Could you check a few things on this model? Use its own coordinates, in mm. Face numbers are marked on the shaded views. A direction names the side the tool comes from. Round coordinates to 2 decimals unless told otherwise and drop trailing zeros. Loops run counter-clockwise (first coordinate to the right, second up) from the corner with the lowest first, then second, coordinate; pieces in that order, holes last. Notation, with made-up numbers: (26, 2) -> (43, 2) arc R15 cw to (43, 27) -> close; hole circle Ø7 at (51, 10). An arc over 180 degrees is marked (long way). One line per item, written item: value.
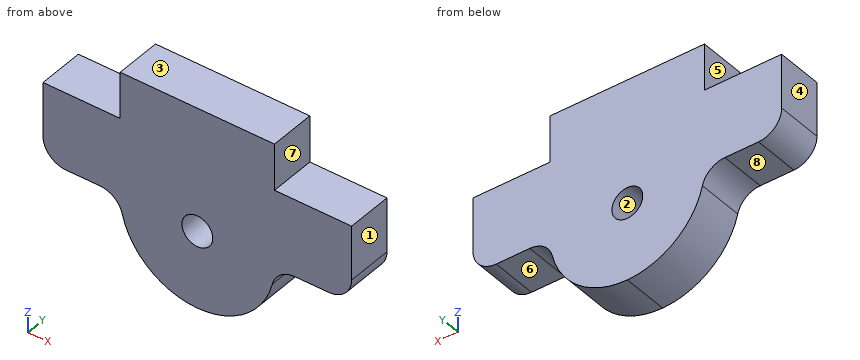
from build123d import *

# Parameters (mm, degrees)
F1_DEPTH = 6
F3_R     = 3
F2_R     = 2
F4_DEPTH = 6.001


with BuildPart() as f1:
    # F0 (on Front) → F1 (new body)
    with BuildSketch(Plane.XZ):
        with BuildLine():
            Line((10, 0), (0, 0))
            Line((0, 0), (-10, 0))
            Line((-10, 0), (-10, -6))
            Line((-10, -6), (-20, -6))
            Line((-20, -6), (-20, -16))
            Line((-20, -16), (-10, -16))
            ThreePointArc((-10, -16), (-7.071068, -23.071068), (0, -26))
            ThreePointArc((0, -26), (7.071068, -23.071068), (10, -16))
            Line((10, -16), (20, -16))
            Line((20, -16), (20, -6))
            Line((20, -6), (10, -6))
            Line((10, -6), (10, 0))
        make_face()
    extrude(amount=F1_DEPTH)

    # F3
    f3_edges = [f1.edges().sort_by_distance(p)[0] for p in [
        (10, -3, -16),
        (-10, -3, -16),
        (20, -3, -16),
        (-20, -3, -16),
    ]]
    fillet(f3_edges, radius=F3_R)

    # F2 (on face) → F4 (cut, through all)
    with BuildSketch(Plane.XZ.offset(6)):
        with Locations((0, -16)):
            Circle(F2_R)
    extrude(amount=-F4_DEPTH, mode=Mode.SUBTRACT)


solid = f1.part
(1) Thinking about a two-plate mould opening in X: for the marked faces 1, 2, 3 and 4, which applies, released by +X, released by -X, zero draft, split by the parting line, or undercut?
Recorded:
face 1: released by +X
face 2: undercut
face 3: zero draft
face 4: released by -X
(2) For the marked faces 5, 6, 7 and 8, which set-ups out of +Z, -Z, +X, -X, +Y, -Y let a thin tool reach every point of the face, with its end or its side?
Recorded:
face 5: +Z, -X, +Y, -Y
face 6: -Z, +X, +Y, -Y
face 7: +Z, +X, +Y, -Y
face 8: -Z, -X, +Y, -Y
(3) If I drill on L1, parallel to X at y = -2.1, z = -17; L2, parallel to Z at x = -15, y = -3.5; L3, parallel to X at y = -2, z = -22.5, over which ranges is the centre line in solid material (lowest first)?
Recorded:
L1: -10.41 to -1.73, 1.73 to 10.41
L2: -16 to -6
L3: -7.6 to 7.6
(4) If we section it at C-C, the plane z = -4.5: Please give me the cut outline in (x, y).
Recorded:
outline: (-10, -6) -> (10, -6) -> (10, 0) -> (-10, 0) -> close
(5) If we section it at B-B, the plane x = -15.5: Please give me the cut outline in (y, z).
Recorded:
outline: (-6, -16) -> (0, -16) -> (0, -6) -> (-6, -6) -> close
(6) I'm going to push flat-ended pins straight in: pin 1 Ø3 at (x, y) = (13, -4) entering from +Z; pin 2 Ø3.5 at (x, y) = (15, -1.5) entering from -Z; pin 3 Ø2.5 at (x, z) = (0, -16) entering from -Y; pin 4 Ø1 at (y, z) = (-1, -5) entering from +X. Where does each tip first touch, or does it pass through?
Recorded:
pin 1: z = -6
pin 2: z = -16
pin 3: through
pin 4: x = 10
(7) If we section it at A-A, the plane y = -5.4: Please give me the cut outline in (x, z), then the cut area to 3 significant figures.
Recorded:
outline: (-20, -13) arc R3 ccw to (-17, -16) -> (-12.65, -16) arc R3 cw to (-9.73, -18.31) arc R10 ccw to (0, -26) arc R10 ccw to (9.73, -18.31) arc R3 cw to (12.65, -16) -> (17, -16) arc R3 ccw to (20, -13) -> (20, -6) -> (10, -6) -> (10, 0) -> (-10, 0) -> (-10, -6) -> (-20, -6) -> close; hole circle Ø4 at (0, -16)
area: 663 mm²
